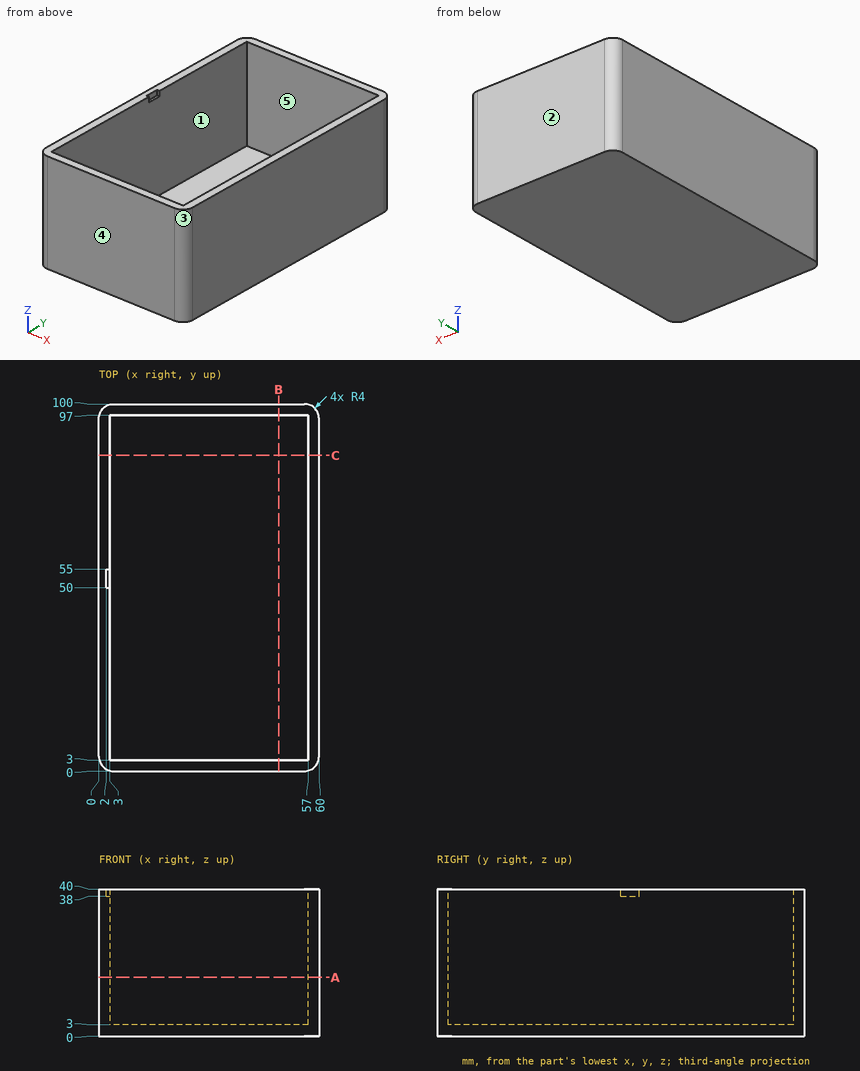
Part print with two shaded views. Sizes in mm from the minimum x, y, z corner. A direction names the side the tool comes from. Coordinates: 2 decimals unless noted, no trailing zeros. Write each loop counter-clockwise with the first axis right and the second up, starting at its lowest first coordinate (ties: lowest second). Pieces come first, ordered by that corner, then holes.
(1) Cut at A-A on z = 16. List the corners of the cut face in (x, y).
(2) 3-axis set-ups, long thin cutter, end or side, ignore diameter. For the marked faces 4 and 5: which of +Z, -Z, +X, -X, +Y, -Y reach the whole face in a straight line?
(3) Mould opens along Y. For the marked faces 1, 2 and 3 say: pulls with the +Y half, pulls with the -Y half, needs draft (parallel to the pull), parting line crosses it, or undercut.
(4) Pin check, flat tips, straight feed: pin 1 Ø1.1 at (x, z) = (2.5, 38.5) entering from -Y; pin 2 Ø1.1 at (x, z) = (2.5, 38.5) entering from +Y. Stop position of each tip, or through.
(5) Drill centre lines: line 1 (X direction, y = 27, z = 5); line 2 (Y direction, x = 49.5, z = 12); line 3 (Z direction, x = 47.5, y = 80). Where is each one in solid material? Low to high.
(6) Cut at C-C on y = 86. List the corners of the cut face in (x, z).
(7) Cut at B-B on x = 49. List the corners of the cut face in (y, z), and give its area (3 significant figures).
Working result:
1. outline: (0, 4) arc R4 ccw to (4, 0) - (56, 0) arc R4 ccw to (60, 4) - (60, 96) arc R4 ccw to (56, 100) - (4, 100) arc R4 ccw to (0, 96) - close; hole (3, 3) - (57, 3) - (57, 97) - (3, 97) - close
2. face 4: +Z, -Z, +X, -X, -Y
2. face 5: +Z
3. face 1: undercut
3. face 2: pulls with the +Y half
3. face 3: pulls with the -Y half
4. pin 1: stops at y = 0.11
4. pin 2: stops at y = 99.89
5. line 1: x = 0 to 3, 57 to 60
5. line 2: y = 0 to 3, 97 to 100
5. line 3: z = 0 to 3
6. outline: (0, 0) - (60, 0) - (60, 40) - (57, 40) - (57, 3) - (3, 3) - (3, 40) - (0, 40) - close
7. outline: (0, 0) - (100, 0) - (100, 40) - (97, 40) - (97, 3) - (3, 3) - (3, 40) - (0, 40) - close
7. area: 522 mm2
